Here's how the part is built. I have some questions about the finished solid (model axes, mm). Face numbers are marked on the shaded views. A direction names the side the tool comes from. Give positions to 0.01 mm unless a question says otherwise; leave off trailing zeros. Use one line per item in the form item = value.
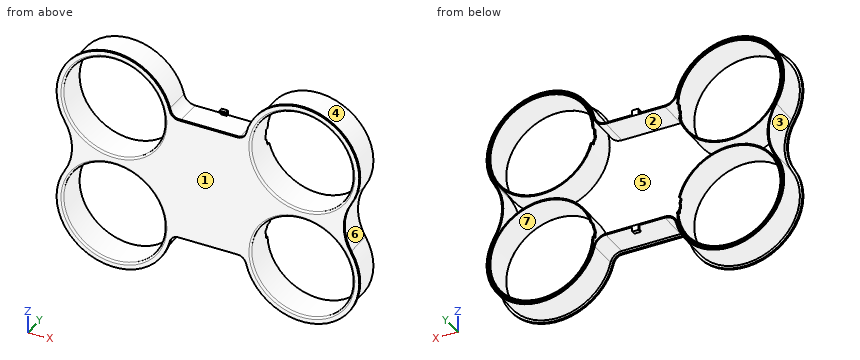
from build123d import *

# Parameters (mm, degrees)
BASE_DEPTH                                  = 25
SKETCH3_R                                   = 40.5
PROPHOLES_DEPTH                             = 25
SHELL2_T                                    = -1
SKETCH4_W                                   = 2
SKETCH4_H                                   = 1.5
HOOKS_DEPTH                                 = 2.5
FILLET1_R                                   = 1.5
ARMHOLES_DEPTH                              = 2.5
ARMDETAILCUT_DEPTH                          = 2.5
ARMDETAILS_AT_THE_SECOND_PLANE_COPY_1_DEPTH = 2.5


with BuildPart() as part:
    # Sketch1 → Base (new body)
    with BuildSketch(Plane(origin=(0, 0, 0), x_dir=(1, 0, 0), z_dir=(0, 1, 0))):
        with BuildLine():
            Line((-23.389824888, 47), (23.389824888, 47))
            ThreePointArc((23.389824888, 47), (28.979355918, 48.946125685), (32.151569193, 53.942857143))
            ThreePointArc((32.151569193, 53.942857143), (90.931692418, 84.277158344), (111.718349922, 21.482352941))
            ThreePointArc((111.718349922, 21.482352941), (105.725511342, 0), (111.718349922, -21.482352941))
            ThreePointArc((111.718349922, -21.482352941), (90.931692418, -84.277158344), (32.151569193, -53.942857143))
            ThreePointArc((32.151569193, -53.942857143), (28.979355918, -48.946125685), (23.389824888, -47))
            Line((23.389824888, -47), (-23.389824888, -47))
            ThreePointArc((-23.389824888, -47), (-28.979355918, -48.946125685), (-32.151569193, -53.942857143))
            ThreePointArc((-32.151569193, -53.942857143), (-90.931692418, -84.277158344), (-111.718349922, -21.482352941))
            ThreePointArc((-111.718349922, -21.482352941), (-105.725511342, 0), (-111.718349922, 21.482352941))
            ThreePointArc((-111.718349922, 21.482352941), (-90.931692418, 84.277158344), (-32.151569193, 53.942857143))
            ThreePointArc((-32.151569193, 53.942857143), (-28.979355918, 48.946125685), (-23.389824888, 47))
        make_face()
    extrude(amount=BASE_DEPTH)

    # Sketch3 → PropHoles (cut)
    with BuildSketch(Plane(origin=(0, 25, 0), x_dir=(1, 0, 0), z_dir=(0, 1, 0))):
        with Locations(Location((74.5, 44, 0), (0, 0, 270))):
            Circle(SKETCH3_R)
        with Locations(Location((74.5, -44, 0), (0, 0, 90))):
            Circle(SKETCH3_R)
        with Locations(Location((-74.5, -44, 0), (0, 0, 270))):
            Circle(SKETCH3_R)
        with Locations(Location((-74.5, 44, 0), (0, 0, 90))):
            Circle(SKETCH3_R)
    extrude(amount=-PROPHOLES_DEPTH, mode=Mode.SUBTRACT)

    # Shell2
    shell2_openings = [part.faces().sort_by_distance(p)[0] for p in [
        (0, 25, 0),
    ]]
    offset(amount=SHELL2_T, openings=shell2_openings, kind=Kind.INTERSECTION)

    # Lip: sweep along a path in Sketch1_2
    with BuildLine(Plane(origin=(0, 0, 0), x_dir=(1, 0, 0), z_dir=(0, 1, 0))) as lip_path:
        Line((-23.389824888, 47), (23.389824888, 47))
        ThreePointArc((23.389824888, 47), (28.979355918, 48.946125685), (32.151569193, 53.942857143))
        ThreePointArc((32.151569193, 53.942857143), (90.931692418, 84.277158344), (111.718349922, 21.482352941))
        ThreePointArc((111.718349922, 21.482352941), (105.725511342, 0), (111.718349922, -21.482352941))
        ThreePointArc((111.718349922, -21.482352941), (90.931692418, -84.277158344), (32.151569193, -53.942857143))
        ThreePointArc((32.151569193, -53.942857143), (28.979355918, -48.946125685), (23.389824888, -47))
        Line((23.389824888, -47), (-23.389824888, -47))
        ThreePointArc((-23.389824888, -47), (-28.979355918, -48.946125685), (-32.151569193, -53.942857143))
        ThreePointArc((-32.151569193, -53.942857143), (-90.931692418, -84.277158344), (-111.718349922, -21.482352941))
        ThreePointArc((-111.718349922, -21.482352941), (-105.725511342, 0), (-111.718349922, 21.482352941))
        ThreePointArc((-111.718349922, 21.482352941), (-90.931692418, 84.277158344), (-32.151569193, 53.942857143))
        ThreePointArc((-32.151569193, 53.942857143), (-28.979355918, 48.946125685), (-23.389824888, 47))
    # Sketch4 → Lip (sweep)
    with BuildSketch(Plane(origin=(0, 0, 0), x_dir=(0, 0, -1), z_dir=(1, 0, 0))):
        with Locations((-48, 0.75)):
            Rectangle(SKETCH4_W, SKETCH4_H)
    sweep(path=lip_path.line)

    # Sketch5 → Hooks (add, symmetric)
    with BuildSketch(Plane(origin=(0, 0, 0), x_dir=(0, 0, -1), z_dir=(1, 0, 0))):
        Polygon((-47, 25), (-50.75, 25), (-50.75, 22), (-49.25, 22), (-49.25, 23.5), (-47, 23.5), align=None)
        Polygon((49.25, 23.5), (47, 23.5), (47, 25), (50.75, 25), (50.75, 22), (49.25, 22), align=None)
    extrude(amount=HOOKS_DEPTH, both=True)

    # Fillet1
    fillet1_edges = [part.edges().sort_by_distance(p)[0] for p in [
        (-74.5, 0, -3.5),
        (-74.5, 0, 3.5),
        (74.5, 0, 84.5),
        (74.5, 0, -84.5),
    ]]
    fillet(fillet1_edges, radius=FILLET1_R)

    # Sketch6 → ArmHoles (cut)
    with BuildSketch(Plane(origin=(0, 25, 0), x_dir=(1, 0, 0), z_dir=(0, 1, 0))):
        with BuildLine():
            Line((74.5, -44), (34.426621288, -33.212307077))
            ThreePointArc((34.426621288, -33.212307077), (33.272270217, -39.25402308), (33.02362118, -45.4))
            Line((33.02362118, -45.4), (74.5, -44))
        make_face()
        with BuildLine():
            Line((74.5, 44), (33.02362118, 45.4))
            ThreePointArc((33.02362118, 45.4), (33.272270217, 39.25402308), (34.426621288, 33.212307077))
            Line((34.426621288, 33.212307077), (74.5, 44))
        make_face()
        with BuildLine():
            Line((-74.5, 44), (-34.426621288, 33.212307077))
            ThreePointArc((-34.426621288, 33.212307077), (-33.272270217, 39.25402308), (-33.02362118, 45.4))
            Line((-33.02362118, 45.4), (-74.5, 44))
        make_face()
        with BuildLine():
            Line((-74.5, -44), (-33.02362118, -45.4))
            ThreePointArc((-33.02362118, -45.4), (-33.272270217, -39.25402308), (-34.426621288, -33.212307077))
            Line((-34.426621288, -33.212307077), (-74.5, -44))
        make_face()
    extrude(amount=-ARMHOLES_DEPTH, mode=Mode.SUBTRACT)

    # Sketch7 → ArmDetailCut (cut)
    with BuildSketch(Plane(origin=(38.732173012, 0, 4.45869807), x_dir=(-0.11436088964892253, 0, 0.9934392718826386), z_dir=(-0.9934392718826385, 0, -0.11436088964892252))):
        with BuildLine():
            Line((36.605160533, 21.5), (33.805160533, 21.5))
            ThreePointArc((33.805160533, 21.5), (33.380896465, 21.675735931), (33.205160533, 22.1))
            Line((33.205160533, 22.1), (33.205160533, 22.5))
            Line((33.205160533, 22.5), (37.205160533, 22.5))
            Line((37.205160533, 22.5), (37.205160533, 22.1))
            ThreePointArc((37.205160533, 22.1), (37.029424602, 21.675735931), (36.605160533, 21.5))
        make_face()
    armdetailcut = extrude(amount=ARMDETAILCUT_DEPTH, mode=Mode.SUBTRACT)

    # ArmDetails: ArmDetailCut across plane
    add(armdetailcut.mirror(Plane.XY), mode=Mode.SUBTRACT)

    # ArmDetails at the second plane: ArmDetailCut across plane
    add(armdetailcut.mirror(Plane(origin=(0, 0, 0), x_dir=(0, 0, 1), z_dir=(1, 0, 0))), mode=Mode.SUBTRACT)

    # ArmDetails at the second plane copy 1 sk → ArmDetails at the second plane copy 1 (cut)
    with BuildSketch(Plane(origin=(-38.732173012, 0, -4.45869807), x_dir=(0.11436088964892253, 0, -0.9934392718826386), z_dir=(0.9934392718826385, 0, 0.11436088964892252))):
        with BuildLine():
            Line((36.605160533, 21.5), (33.805160533, 21.5))
            ThreePointArc((33.805160533, 21.5), (33.380896465, 21.675735931), (33.205160533, 22.1))
            Line((33.205160533, 22.1), (33.205160533, 22.5))
            Line((33.205160533, 22.5), (37.205160533, 22.5))
            Line((37.205160533, 22.5), (37.205160533, 22.1))
            ThreePointArc((37.205160533, 22.1), (37.029424602, 21.675735931), (36.605160533, 21.5))
        make_face()
    extrude(amount=ARMDETAILS_AT_THE_SECOND_PLANE_COPY_1_DEPTH, mode=Mode.SUBTRACT)


solid = part.part
Q1. Thinking about a two-plate mould opening in X: for the marked faces 1, 2, 3 and 4, which applies, +X half, -X half, draft (parallel to the pull), parting line (faces both ways), or undercut?
Found:
face_1 = draft
face_2 = undercut
face_3 = -X half
face_4 = undercut
Q2. On a 3-axis mill with a long thin cutter (end or side, diameter ignored), from which of +Z, -Z, +X, -X, +Y, -Y can I reach the whole of each face in a straight line? I mean the marked faces 5, 6 and 7. Say none if no direction works.
Found:
face_5 = +Y
face_6 = +X, +Y
face_7 = +Y, -Y
Q3. I need wall thicknesses on L1, parallel to Z at x = -72.5, y = 15; L2, parallel to X at y = 9, z = -44; L3, parallel to Z at x = 82.5, y = 17.75. Which ranges of each line are inside material? Lowest first, please.
Found:
L1 = -87.45 to -86.45, -85.45 to -84.45, -3.55 to -2.55, 2.55 to 3.55, 84.45 to 85.45, 86.45 to 87.45
L2 = -118 to -117, -116 to -115, -34 to -33, 33 to 34, 115 to 116, 117 to 118
L3 = -86.76 to -85.74, -84.72 to -83.7, -4.3 to -3.28, 3.28 to 4.3, 83.7 to 84.72, 85.74 to 86.76
Q4. I'm going to push flat-ended pins straight in: pin 1 Ø3.5 at (y, z) = (23, 48.5) entering from -X; pin 2 Ø0.9 at (y, z) = (24, 48.5) entering from +X; pin 3 Ø1.5 at (y, z) = (18, 4) entering from +X. Where does each tip first touch, or does it pass through?
Found:
pin_1 = -117.91
pin_2 = 117.81
pin_3 = 106
Q5. I want a section at A-A on y = 7.5. State how many separate pieces and enclosed holes the cut face has, then the cut area to 3 significant figures.
Found:
separate_pieces = 5
enclosed_holes = 5
area = 1,860 mm²
